from build123d import *

# Parameters (mm, degrees)
SKETCH4_W          = 50.332275622
SKETCH4_H          = 47.611612075
CUT_EXTRUDE1_DEPTH = 10


with BuildPart() as part:
    # Sketch1 → Revolve3 (revolve)
    with BuildSketch(Plane.XY, mode=Mode.PRIVATE) as revolve3_sk:
        Polygon((0, 150), (-41.5, 0), (-33, 0), (-33, 2), (-38.871533471, 2), (0, 142.499518572), align=None)
    revolve(revolve3_sk.sketch.rotate(Axis((0, 2, 0), (0, 1, 0)), 270), axis=Axis((0, 2, 0), (0, 1, 0)))

    # Sketch2 → Revolve6 (revolve)
    with BuildSketch(Plane.XY, mode=Mode.PRIVATE) as revolve6_sk:
        Polygon((33, 30.722891566), (33, -50), (38, -50), (38, 0), (41.5, 0), align=None)
    revolve(revolve6_sk.sketch.rotate(Axis((0, 0, 0), (0, -1, 0)), 270), axis=Axis((0, 0, 0), (0, -1, 0)))

    # Sketch4 → Cut-Extrude1 (cut)
    with BuildSketch(Plane(origin=(0, 149.9, 0), x_dir=(1, 0, 0), z_dir=(0, 1, 0))):
        with Locations((0.291499666, 1.846164549)):
            Rectangle(SKETCH4_W, SKETCH4_H)
    extrude(amount=CUT_EXTRUDE1_DEPTH, mode=Mode.SUBTRACT)


solid = part.part
The listing builds one solid part. Answer for the finished solid, in the listing's coordinates (mm). Give positions to 0.01 mm unless a question says otherwise; leave off trailing zeros. Write each loop counter-clockwise with the first axis right and the second up, starting at its lowest first coordinate (ties: lowest second). Pieces come first, ordered by that corner, then holes.
Item 1: Find the intervals of material crossed by line 1 along X through (y, z) = (-3, 0); line 2 along X through (y, z) = (89, -8.5); line 3 along Z through (x, y) = (-6.5, 71), in increasing order.
Item 2: Determine the mould class of faces 1 (the cylindrical face through (-32.215, -13.901, 7.154)), 2 (the flat face through (34, 0, -18)), 3 (the cylindrical face through (-23.122, -24.65, 30.156)) for opening direction Z: released by +Z, released by -Z, zero draft, split by the parting line, or undercut.
Item 3: Section A-A, the plane y = 70.5 is taken. Write down the section's boundary in (x, z) (3 decimals).
Item 4: Section B-B, the plane y = 37 is taken. Write down the section's boundary in (x, z).
Item 5: Flat-ended cylindrical pins translate along their axes: P1, Ø2, axis at x = -31, z = -26, coming from the -Y side; P2, Ø3, axis at y = 18, z = -13.5, coming from the +X side; P3, Ø2, axis at x = -20, y = -11, coming from the +Z side. Find the tip coordinate at first contact, or state that the pin passes through.
Completed:
1. line 1: x = -38 to -33, 33 to 38
1. line 2: x = -14.58 to -12.12, 12.12 to 14.58
1. line 3: z = -20.87 to -18.68, 18.68 to 20.87
2. face 1: undercut
2. face 2: zero draft
2. face 3: split by the parting line
3. outline: circle Ø43.99 at (0, 0); hole circle Ø39.84 at (0, 0)
4. outline: circle Ø62.53 at (0, 0); hole circle Ø58.38 at (0, 0)
5. P1: stops at y = 0
5. P2: stops at x = 34.65
5. P3: stops at z = 32.91
